from build123d import *

# Parameters (mm, degrees)
F0_W     = 63.5
F0_H     = 63.5
F0_R     = 28.575
F1_DEPTH = 7.9375
F3_DEPTH = 25.4


# Not quite as in the source:
# - a length typed as a fraction of an inch, garbled in the dataset ("3 / 203.2 mm" for 3/8 in), is restored


with BuildPart() as f1:
    # F0 (on Front) → F1 (new body)
    with BuildSketch(Plane.XZ):
        Rectangle(F0_W, F0_H)
        Circle(F0_R, mode=Mode.SUBTRACT)
    extrude(amount=F1_DEPTH)

    # F2 (on face) → F3 (cut)
    with BuildSketch(Plane.XZ.offset(7.9375)):
        with BuildLine():
            ThreePointArc((-22.8203125, -25.4), (-27.2241145246, -23.5758854754), (-25.4, -27.9796875))
            ThreePointArc((-25.4, -27.9796875), (-23.5758854754, -27.2241145246), (-22.8203125, -25.4))
        make_face()
    extrude(amount=-F3_DEPTH, mode=Mode.SUBTRACT)


solid = f1.part
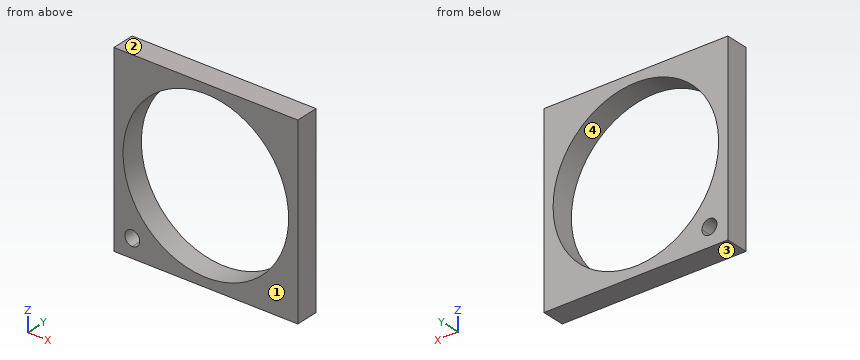
Geometry check sheet. Reference: the model listing, model coordinates, mm. Face numbers are marked on the shaded views. Give positions to 0.01 mm unless a question says otherwise; leave off trailing zeros. Write each loop counter-clockwise with the first axis right and the second up, starting at its lowest first coordinate (ties: lowest second). Pieces come first, ordered by that corner, then holes. Notation, with made-up numbers: (46, 71) - (53, 71) arc R14 cw to (53, 91) - close; hole circle Ø4 at (59.5, 78.25). An arc over 180 degrees is marked (long way). Put each result on its own line as item: value.
1. Draft check along Z on the marked faces 1, 2, 3 and 4. Enter one of: +Z half, -Z half, draft (parallel to the pull), parting line (faces both ways), or undercut.
Ans:
face 1: draft
face 2: +Z half
face 3: -Z half
face 4: undercut
2. Thickness scan on line 1 (Z direction, x = 0, y = -1.75) (3 decimals); line 2 (X direction, y = -2.75, z = -25.4); line 3 (X direction, y = -1, z = 19.5). Record the ranges inside material, lowest first.
Ans:
line 1: z = -31.75 to -28.575, 28.575 to 31.75
line 2: x = -31.75 to -27.98, -22.82 to -13.09, 13.09 to 31.75
line 3: x = -31.75 to -20.89, 20.89 to 31.75
3. Sectioned sample at C-C, the plane y = -7. Enter the section's corners in (x, z) (3 decimals).
Ans:
outline: (-31.75, -31.75) - (31.75, -31.75) - (31.75, 31.75) - (-31.75, 31.75) - close; hole circle Ø57.15 at (0, 0); hole circle Ø5.159 at (-25.4, -25.4)
4. Go/stop test with a flat-tipped pin: pin 1 (6.5 mm diameter, centred on x = -25.4, z = -25.4, fed in from +Y). Record where the tip stops, or that it passes through.
Ans:
pin 1: stops at y = 0
